Read the model definition and answer for the solid it produces. Units are mm, in the model's axes. Face numbers are marked on the shaded views. Coordinates: 2 decimals unless noted, no trailing zeros. Order: outer loops, then holes, each group sorted by start corner. A loop starts at its lowest first (then second) coordinate and runs counter-clockwise, first axis right, second up. Notation, with made-up numbers: (81, 30.5) -> (135, 30.5) arc R25 cw to (135, 65.5) -> close; hole circle Ø8 at (-7.75, 50.25). An arc over 180 degrees is marked (long way). Use CSV: the item, a comma, the result in double quotes.
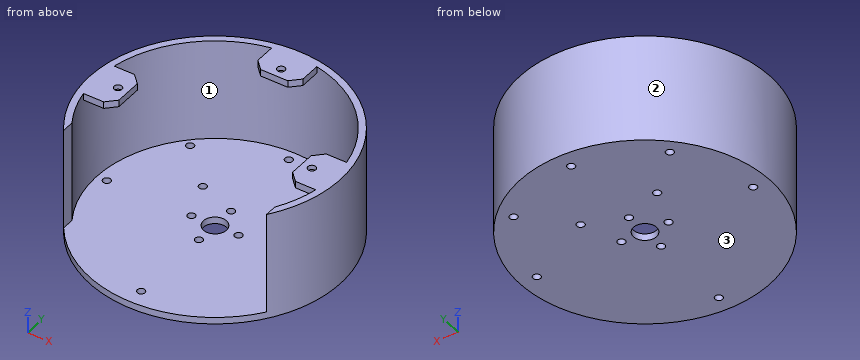
```python
from build123d import *

# Parameters (mm, degrees)
SKETCH1_R           = 55.5
SKETCH1_R_2         = 52.5
BOSS_EXTRUDE1_DEPTH = 45
BOSS_EXTRUDE2_START = 3
SKETCH2_R           = 55.5
SKETCH2_R_2         = 5.1
SKETCH2_R_3         = 1.7
BOSS_EXTRUDE2_DEPTH = 3
SKETCH3_W           = 90
SKETCH3_H           = 75.046354864
CUT_EXTRUDE1_DEPTH  = 91.4737531
BOSS_EXTRUDE3_START = -3
SKETCH4_R           = 1.75
BOSS_EXTRUDE3_DEPTH = 3
CHAMFER1_SIZE       = 4
SKETCH8_R           = 1.7
CUT_EXTRUDE2_DEPTH  = 10
SKETCH9_R           = 3.25
CUT_EXTRUDE3_DEPTH  = 1


with BuildPart() as part:
    # Sketch1 → Boss-Extrude1 (new body)
    with BuildSketch(Plane.XY):
        with Locations(Location((0, 0, 0), (0, 0, 180))):
            Circle(SKETCH1_R)
        with Locations(Location((0, 0, 0), (0, 0, 180))):
            Circle(SKETCH1_R_2, mode=Mode.SUBTRACT)
    extrude(amount=BOSS_EXTRUDE1_DEPTH)

    # Sketch2 → Boss-Extrude2 (add)
    with BuildSketch(Plane(origin=(0, 0, 0), x_dir=(-1, 0, 0), z_dir=(0, 0, -1)).offset(BOSS_EXTRUDE2_START)):
        Circle(SKETCH2_R)
        Circle(SKETCH2_R_2, mode=Mode.SUBTRACT)
        with Locations((-10.45, 0)):
            Circle(SKETCH2_R_3, mode=Mode.SUBTRACT)
        with Locations((10.45, 0)):
            Circle(SKETCH2_R_3, mode=Mode.SUBTRACT)
        with Locations((0, 10.45)):
            Circle(SKETCH2_R_3, mode=Mode.SUBTRACT)
        with Locations((0, -10.45)):
            Circle(SKETCH2_R_3, mode=Mode.SUBTRACT)
    extrude(amount=-BOSS_EXTRUDE2_DEPTH)

    # Sketch3 → Cut-Extrude1 (cut, through all)
    with BuildSketch(Plane(origin=(0, 0, 0), x_dir=(1, 0, 0), z_dir=(0, 1, 0))):
        with Locations((0, -37.523177432)):
            Rectangle(SKETCH3_W, SKETCH3_H)
    extrude(amount=-CUT_EXTRUDE1_DEPTH, mode=Mode.SUBTRACT)

    # Sketch4 → Boss-Extrude3 (add)
    # profile 1 of 3: a face of its own
    with BuildSketch(Plane.XY.offset(45).offset(BOSS_EXTRUDE3_START)):
        with BuildLine():
            Line((51.53882032, -10), (38.53882032, -10))
            Line((38.53882032, -10), (38.53882032, 10))
            Line((38.53882032, 10), (51.53882032, 10))
            ThreePointArc((51.53882032, 10), (52.5, 0), (51.53882032, -10))
        make_face()
        with Locations((43, 0)):
            Circle(SKETCH4_R, mode=Mode.SUBTRACT)
    # profile 2 of 3: a face of its own
    with BuildSketch(Plane.XY.offset(45).offset(BOSS_EXTRUDE3_START)):
        with BuildLine():
            Line((-51.53882032, 10), (-38.53882032, 10))
            Line((-38.53882032, 10), (-38.53882032, -10))
            Line((-38.53882032, -10), (-51.53882032, -10))
            ThreePointArc((-51.53882032, -10), (-52.5, 0), (-51.53882032, 10))
        make_face()
        with Locations((-43, 0)):
            Circle(SKETCH4_R, mode=Mode.SUBTRACT)
    # profile 3 of 3: a face of its own
    with BuildSketch(Plane.XY.offset(45).offset(BOSS_EXTRUDE3_START)):
        with BuildLine():
            Line((10, 51.53882032), (10, 38.53882032))
            Line((10, 38.53882032), (-10, 38.53882032))
            Line((-10, 38.53882032), (-10, 51.53882032))
            ThreePointArc((-10, 51.53882032), (0, 52.5), (10, 51.53882032))
        make_face()
        with Locations((0, 43)):
            Circle(SKETCH4_R, mode=Mode.SUBTRACT)
    extrude(amount=BOSS_EXTRUDE3_DEPTH)

    # Chamfer1
    chamfer1_edges = [part.edges().sort_by_distance(p)[0] for p in [
        (38.53882032, -10, 43.5),
        (38.53882032, 10, 43.5),
        (-38.53882032, 10, 43.5),
        (-38.53882032, -10, 43.5),
        (10, 38.53882032, 43.5),
        (-10, 38.53882032, 43.5),
    ]]
    chamfer(chamfer1_edges, length=CHAMFER1_SIZE)

    # Sketch8 → Cut-Extrude2 (cut)
    with BuildSketch(Plane(origin=(0, 0, -3), x_dir=(-1, 0, 0), z_dir=(0, 0, -1))):
        with Locations((34.648232278, 34.648232278)):
            Circle(SKETCH8_R)
        with Locations((16.970562748, 16.970562748)):
            Circle(SKETCH8_R)
        with Locations((-16.970562748, 16.970562748)):
            Circle(SKETCH8_R)
        with Locations((-34.648232278, 34.648232278)):
            Circle(SKETCH8_R)
        with Locations((0, -48)):
            Circle(SKETCH8_R)
        with Locations((-48, 0)):
            Circle(SKETCH8_R)
        with Locations((0, 48)):
            Circle(SKETCH8_R)
        with Locations((48, 0)):
            Circle(SKETCH8_R)
    extrude(amount=-CUT_EXTRUDE2_DEPTH, mode=Mode.SUBTRACT)

    # Sketch9 → Cut-Extrude3 (cut)
    with BuildSketch(Plane(origin=(0, 0, 42), x_dir=(-1, 0, 0), z_dir=(0, 0, -1))):
        with Locations((-43, 0)):
            Circle(SKETCH9_R)
        with Locations((0, 43)):
            Circle(SKETCH9_R)
        with Locations((43, 0)):
            Circle(SKETCH9_R)
    extrude(amount=-CUT_EXTRUDE3_DEPTH, mode=Mode.SUBTRACT)


solid = part.part
```
Item 1: Find section C-C, the plane z = 19. Give the vertices of the cut face in (x, y).
Return value:
outline,"(-45, -32.48) -> (-45, -27.04) arc R52.5 cw (long way) to (45, -27.04) -> (45, -32.48) arc R55.5 ccw (long way) to start"
Item 2: Find section A-A, the plane y = 48. Give the vertices of the cut face in (x, z).
Return value:
outline,"(-27.86, -3) -> (-1.7, -3) -> (-1.7, 0) -> (-21.27, 0) -> (-21.27, 45) -> (-27.86, 45) -> close; (-10, 42) -> (10, 42) -> (10, 45) -> (-10, 45) -> close; (1.7, -3) -> (27.86, -3) -> (27.86, 45) -> (21.27, 45) -> (21.27, 0) -> (1.7, 0) -> close"
Item 3: Find section D-D, the plane x = 24. Give the vertices of the cut face in (y, z), then the cut area to 3 significant figures.
Return value:
outline,"(-50.04, -3) -> (50.04, -3) -> (50.04, 45) -> (46.69, 45) -> (46.69, 0) -> (-50.04, 0) -> close"
area,"451 mm^2"
Item 4: The mould has two halves that part along X. Classify the marked faces 1, 2 and 3: +X half, -X half, draft (parallel to the pull), parting line (faces both ways), or undercut.
Return value:
face 1,"undercut"
face 2,"parting line"
face 3,"draft"
Item 5: Each of these flat-tipped pins is pushed along its axis until it touches: P1, Ø1, axis at x = 16.5, z = 19.5, coming from the +Y side; P2, Ø3, axis at x = -43, y = 0, coming from the +Z side; P3, Ø2.5, axis at y = 46.5, z = 43, coming from the -X side. Where does it stop, or does it pass through?
Return value:
P1,"stops at y = 53.14"
P2,"stops at z = 0"
P3,"stops at x = -32.14"
Item 6: Find section B-B, the plane y = -48. Give the vertices of the cut face in (x, z).
Return value:
outline,"(-27.86, -3) -> (-1.7, -3) -> (-1.7, 0) -> (-27.86, 0) -> close; (1.7, -3) -> (27.86, -3) -> (27.86, 0) -> (1.7, 0) -> close"
Item 7: Straight lines are drawn through the part: line 1 along Z through (x, y) = (-14.5, 35); line 2 along Y through (x, z) = (43, 42.35); line 3 along X through (y, z) = (36, 21). For each, find the intervals that lie inside material, in ascending order.
Return value:
line 1,"z = -3 to 0"
line 2,"y = -10 to -3.25, 3.25 to 10, 30.12 to 35.09"
line 3,"x = -42.24 to -38.21, 38.21 to 42.24"
